Verification items for the finished model (mm, model axes). A direction names the side the tool comes from. Round coordinates to 2 decimals unless told otherwise and drop trailing zeros. Write each loop counter-clockwise with the first axis right and the second up, starting at its lowest first coordinate (ties: lowest second). Pieces come first, ordered by that corner, then holes. Notation, with made-up numbers: M 57.25,-29 L 113.25,-29 A33 cw 113.25,1 Z; hole C 71,38 d7. An arc over 180 degrees is marked long. Answer in a Markdown table with one row per item. Add a question column.
1. Sectioned sample at A-A on x = 71. Record the cut outline in (y, z).
2. Sectioned sample at C-C on x = -16. Record the cut outline in (y, z), plus the area to 3 significant figures.
3. Material ranges on probe 1 along Y at (x, z) = (-71, 3); probe 2 along X at (y, z) = (-3, 1.25); probe 3 along Y at (x, z) = (23, 4.5), recorded low to high.
4. Set-up check for faces 1 (the flat face through (-1, 34, 3)), 2 (the flat face through (0, 24, 3)): record each of +Z, -Z, +X, -X, +Y, -Y from which the full face is reachable in a straight line by a thin tool's end or side.
5. Sectioned sample at D-D on z = 2.25. Count the separate pieces of the cut face and the enclosed holes in it, plus the area to 3 significant figures.
6. Go/stop test with flat-tipped pins: pin 1 Ø8 at (x, y) = (41, 8) entering from -Z; pin 2 Ø3 at (x, z) = (-83.5, 3.5) entering from -Y. Record where each tip stops, or that it passes through.
7. Draft check along X on faces 3 (the cylindrical face through (80.849, -20.916, 3.219)), 4 (the cylindrical face through (118.07, 19.4, 3.22)), 5 (the cylindrical face through (-118.12, -19.33, 3.22)). Enter one of: pulls with the +X half, pulls with the -X half, needs draft (parallel to the pull), parting line crosses it, or undercut.
8. Sectioned sample at B-B on y = 29. Record the cut outline in (x, z).
```python
from build123d import *

# Parameters (mm, degrees)
BOSS_EXTRUDE1_DEPTH      = 6.35
M3_CLEARANCE_HOLE1_D     = 3.2
M3_CLEARANCE_HOLE1_DEPTH = 95.7
M3_CLEARANCE_HOLE1_TIP   = 0.96137699
FILLET1_R                = 5
FILLET2_R                = 15
CUT_EXTRUDE1_DEPTH       = 124.924664615
SKETCH6_W                = 10
SKETCH6_H                = 48
BOSS_EXTRUDE2_DEPTH      = 6.35
EXTRUDE_THIN1_DEPTH      = 6.35
F_4_0_REAMED_D           = 4
MIRROR3_COPY_1_D         = 4
FILLET3_R                = 5


with BuildPart() as part:
    # Sketch1 → Boss-Extrude1 (new body)
    with BuildSketch(Plane.XY):
        Polygon((80.535316128, 34), (119, 20), (119, -20), (80.535316128, -34), (-80.535316128, -34), (-119, -20), (-119, 20), (-80.535316128, 34), align=None)
    extrude(amount=BOSS_EXTRUDE1_DEPTH)

    # M3 Clearance Hole1
    with Locations(Plane(origin=(0, 0, 0), x_dir=(1, 0, 0), z_dir=(0, 0, -1))):
        with Locations((115.825, -12.5), (115.825, 12.5), (-115.825, 12.5), (-115.825, -12.5)):
            Hole(M3_CLEARANCE_HOLE1_D / 2, depth=M3_CLEARANCE_HOLE1_DEPTH)
            with Locations((0, 0, -(M3_CLEARANCE_HOLE1_DEPTH + M3_CLEARANCE_HOLE1_TIP / 2))):  # 118° drill point
                Cone(0, M3_CLEARANCE_HOLE1_D / 2, M3_CLEARANCE_HOLE1_TIP, mode=Mode.SUBTRACT)

    # Fillet1
    fillet1_edges = [part.edges().sort_by_distance(p)[0] for p in [
        (119, -20, 3.175),
        (-119, -20, 3.175),
        (-119, 20, 3.175),
        (119, 20, 3.175),
    ]]
    fillet(fillet1_edges, radius=FILLET1_R)

    # Fillet2
    fillet2_edges = [part.edges().sort_by_distance(p)[0] for p in [
        (80.535316128, -34, 3.175),
        (-80.535316128, -34, 3.175),
        (-80.535316128, 34, 3.175),
        (80.535316128, 34, 3.175),
    ]]
    fillet(fillet2_edges, radius=FILLET2_R)

    # Sketch5 → Cut-Extrude1 (cut, through all)
    with BuildSketch(Plane(origin=(0, 0, 0), x_dir=(-1, 0, 0), z_dir=(0, 0, -1))):
        Polygon((-78.772046321, 24), (-109, 12.997924618), (-109, -12.997924618), (-78.772046321, -24), (78.772046321, -24), (109, -12.997924618), (109, 12.997924618), (78.772046321, 24), align=None)
    extrude(amount=-CUT_EXTRUDE1_DEPTH, mode=Mode.SUBTRACT)

    # Sketch6 → Boss-Extrude2 (add)
    with BuildSketch(Plane(origin=(0, 0, 0), x_dir=(-1, 0, 0), z_dir=(0, 0, -1))):
        with Locations((-73.772046321, 0)):
            Rectangle(SKETCH6_W, SKETCH6_H)
        with Locations((73.772046321, 0)):
            Rectangle(SKETCH6_W, SKETCH6_H)
    extrude(amount=-BOSS_EXTRUDE2_DEPTH)

    # Sketch7 → Extrude-Thin1 (add)
    with BuildSketch(Plane(origin=(0, 0, 0), x_dir=(-1, 0, 0), z_dir=(0, 0, -1))):
        Polygon((67.124588801, 28.720792701), (-70.41950384, -19.279207299), (-67.124588801, -28.720792701), (70.41950384, 19.279207299), align=None)
    extrude_thin1 = extrude(amount=-EXTRUDE_THIN1_DEPTH)

    # Mirror1: Extrude-Thin1 across plane
    add(extrude_thin1.mirror(Plane(origin=(0, 0, 0), x_dir=(0, 0, 1), z_dir=(1, 0, 0))))

    # Ø4.0 Reamed (through all)
    with Locations(Plane(origin=(0, 0, 0), x_dir=(-1, 0, 0), z_dir=(0, 0, -1))):
        with Locations((-71, -29), (-63, -29), (-71, -21)):
            f_4_0_reamed = Hole(F_4_0_REAMED_D / 2)

    # Mirror2: Ø4.0 Reamed across plane
    add(f_4_0_reamed.mirror(Plane(origin=(0, 0, 0), x_dir=(0, 0, 1), z_dir=(1, 0, 0))), mode=Mode.SUBTRACT)

    # Mirror3: Ø4.0 Reamed across plane
    add(f_4_0_reamed.mirror(Plane.ZX), mode=Mode.SUBTRACT)

    # Mirror3 copy 1 (through all)
    with Locations(Plane(origin=(0, 0, 0), x_dir=(1, 0, 0), z_dir=(0, 0, -1))):
        with Locations((-71, -29), (-63, -29), (-71, -21)):
            Hole(MIRROR3_COPY_1_D / 2)

    # Fillet3
    fillet3_edges = [part.edges().sort_by_distance(p)[0] for p in [
        (-78.772046321, -24, 3.175),
        (78.772046321, -24, 3.175),
        (109, -12.997924618, 3.175),
        (109, 12.997924618, 3.175),
        (78.772046321, 24, 3.175),
        (-78.772046321, 24, 3.175),
        (-109, 12.997924618, 3.175),
        (-109, -12.997924618, 3.175),
        (-68.772046321, 18.704279221, 3.175),
        (68.772046321, -18.704279221, 3.175),
        (53.597148206, -24, 3.175),
        (-53.597148206, 24, 3.175),
        (0, -5.295720779, 3.175),
        (-15.174898114, 0, 3.175),
        (-68.772046321, -18.704279221, 3.175),
        (53.597148206, 24, 3.175),
        (0, 5.295720779, 3.175),
        (-53.597148206, -24, 3.175),
        (68.772046321, 18.704279221, 3.175),
        (15.174898114, 0, 3.175),
    ]]
    fillet(fillet3_edges, radius=FILLET3_R)


solid = part.part
```
Geometry check:
| question | item | result |
|---|---|---|
| 1 | outline | M -34,0 L -31,0 L -31,6.35 L -34,6.35 Z; M -27,0 L -23,0 L -23,6.35 L -27,6.35 Z; M -19,0 L 19,0 L 19,6.35 L -19,6.35 Z; M 23,0 L 27,0 L 27,6.35 L 23,6.35 Z; M 31,0 L 34,0 L 34,6.35 L 31,6.35 Z |
| 2 | outline | M -34,0 L -24,0 L -24,6.35 L -34,6.35 Z; M -10.88,0 L 10.88,0 L 10.88,6.35 L -10.88,6.35 Z; M 24,0 L 34,0 L 34,6.35 L 24,6.35 Z |
| 2 | area | 265 mm2 |
| 3 | probe 1 | y = -34 to -31, -27 to -23, -19 to 19, 23 to 27, 31 to 34 |
| 3 | probe 2 | x = -119 to -109, -78.77 to -68.77, -26.35 to 26.35, 68.77 to 78.77, 109 to 119 |
| 3 | probe 3 | y = -34 to -24, -13.32 to 13.32, 24 to 34 |
| 4 | face 1 | +Z, -Z, +X, -X, +Y |
| 4 | face 2 | +Z, -Z |
| 5 | separate pieces | 1 |
| 5 | enclosed holes | 22 |
| 5 | area | 9,300 mm2 |
| 6 | pin 1 | stops at z = 0 |
| 6 | pin 2 | stops at y = -33.43 |
| 7 | face 3 | undercut |
| 7 | face 4 | pulls with the +X half |
| 7 | face 5 | pulls with the -X half |
| 8 | outline | M -94.27,0 L -73,0 L -73,6.35 L -94.27,6.35 Z; M -69,0 L -65,0 L -65,6.35 L -69,6.35 Z; M -61,0 L 61,0 L 61,6.35 L -61,6.35 Z; M 65,0 L 69,0 L 69,6.35 L 65,6.35 Z; M 73,0 L 94.27,0 L 94.27,6.35 L 73,6.35 Z |
